```python
from build123d import *

# Parameters (mm, degrees)
SKETCH1_R           = 75
BOSS_EXTRUDE1_DEPTH = 20
BOSS_EXTRUDE2_DEPTH = 7.5
BOSS_EXTRUDE3_START = 7.5
SKETCH2_4_R         = 2.25
BOSS_EXTRUDE3_DEPTH = 20
BOSS_EXTRUDE4_START = -22.5
SKETCH2_5_R         = 2.25
BOSS_EXTRUDE4_DEPTH = 15


with BuildPart() as part:
    # Sketch1 → Boss-Extrude1 (new body)
    with BuildSketch(Plane(origin=(0, 0, 0), x_dir=(1, 0, 0), z_dir=(0, 1, 0))):
        with Locations(Location((0, 0, 0), (0, 0, 270))):
            Circle(SKETCH1_R)
    extrude(amount=BOSS_EXTRUDE1_DEPTH)

    # Sketch2 → Boss-Extrude2 (add, symmetric)
    with BuildSketch(Plane.XY):
        Polygon((75, 20), (-75, 20), (-117.25, 55), (0, 55), (75, 60), align=None)
    extrude(amount=BOSS_EXTRUDE2_DEPTH, both=True)

    # Sketch2<4> → Boss-Extrude3 (add)
    # profile 1 of 2: a face of its own
    with BuildSketch(Plane.XY.offset(BOSS_EXTRUDE3_START)):
        Polygon((-75, 20), (75, 20), (75, 60), (0, 55), (-117.25, 55), align=None)
    # profile 2 of 2: a face of its own
    with BuildSketch(Plane.XY.offset(BOSS_EXTRUDE3_START)):
        Polygon((0, 55), (75, 60), (-65, 90), (-65, 170), (-117.25, 170), (-117.25, 55), align=None)
        with Locations((-95, 80)):
            Circle(SKETCH2_4_R, mode=Mode.SUBTRACT)
        with Locations((-95, 150)):
            Circle(SKETCH2_4_R, mode=Mode.SUBTRACT)
    extrude(amount=BOSS_EXTRUDE3_DEPTH)

    # Sketch2<5> → Boss-Extrude4 (add)
    with BuildSketch(Plane.XY.offset(BOSS_EXTRUDE4_START)):
        Polygon((75, 20), (-75, 20), (-117.25, 55), (-117.25, 170), (-65, 170), (-65, 90), (75, 60), align=None)
        with Locations((-95, 150)):
            Circle(SKETCH2_5_R, mode=Mode.SUBTRACT)
        with Locations((-95, 80)):
            Circle(SKETCH2_5_R, mode=Mode.SUBTRACT)
    extrude(amount=BOSS_EXTRUDE4_DEPTH)


solid = part.part
```
Here's how the part is built. I have some questions about the finished solid (model axes, mm). A direction names the side the tool comes from. Give positions to 0.01 mm unless a question says otherwise; leave off trailing zeros. Write each loop counter-clockwise with the first axis right and the second up, starting at its lowest first coordinate (ties: lowest second). Pieces come first, ordered by that corner, then holes.
(1) Will these pins go through, and if not, where does the flat tip stop? pin 1 (1.5 mm diameter, centred on x = -63.5, y = 72, fed in from +Z); pin 2 (6 mm diameter, centred on y = 120.5, z = 15, fed in from +X); pin 3 (4 mm diameter, centred on x = -85.5, y = 135.5, fed in from -Z).
Output values:
pin 1: stops at z = 27.5
pin 2: stops at x = -65
pin 3: stops at z = -22.5
(2) Imagine slicing it at D-D, the plane x = -49. Write out the boundary of the cut face in (y, z).
Output values:
outline: (0, -56.78) - (20, -56.78) - (20, -22.5) - (86.57, -22.5) - (86.57, -7.5) - (55, -7.5) - (55, 7.5) - (86.57, 7.5) - (86.57, 27.5) - (20, 27.5) - (20, 56.78) - (0, 56.78) - close
(3) If I drill on L1, parallel to Z at x = -54.5, y = 77; L2, parallel to X at y = 150, z = -13.5; L3, parallel to Y at x = -95, z = 12, over which ranges is the centre line in solid material (lowest first)?
Output values:
L1: z = -22.5 to -7.5, 7.5 to 27.5
L2: x = -117.25 to -97.25, -92.75 to -65
L3: y = 36.57 to 77.75, 82.25 to 147.75, 152.25 to 170
(4) On a 3-axis mill with a long thin cutter (end or side, diameter ignored), from which of +Z, -Z, +X, -X, +Y, -Y can I reach the whole of each face in a straight line? I mean faces 1 (the face through (73, 20, 20)), 2 (the face through (-65, 131, -15)), 3 (the face through (1, 20, 46)), 4 (the face through (-45.636, 9.86, -59.517)), 5 (the face through (-41, 79, -22.5)). Say none if no direction works.
Output values:
face 1: +Z, +X, -Y
face 2: +Z, -Z, +X, +Y
face 3: +Z, +X, -X, +Y
face 4: -Y
face 5: -Z, +X, -X, +Y
(5) Imagine slicing it at C-C, the plane y = 41. Write out the boundary of the cut face in (x, z).
Output values:
outline: (-100.35, -22.5) - (75, -22.5) - (75, 27.5) - (-100.35, 27.5) - close
(6) Imagine slicing it at B-B, the plane z = 23. Write out the boundary of the cut face in (x, y), and give its area (3 significant figures).
Output values:
outline: (-117.25, 55) - (-75, 20) - (-71.39, 20) - (-71.39, 0) - (71.39, 0) - (71.39, 20) - (75, 20) - (75, 60) - (-65, 90) - (-65, 170) - (-117.25, 170) - close; hole circle Ø4.5 at (-95, 80); hole circle Ø4.5 at (-95, 150)
area: 17,600 mm2
(7) Thinking about a two-plate mould opening in Y: for faces 6 (the face through (-92.92, 149.14, 17.36)), 7 (the face through (-71, 104, -7.5)), 8 (the face through (-92.92, 79.14, 17.36)), 9 (the face through (5.98, 74.79, 17.36)), which applies, pulls with the +Y half, pulls with the -Y half, needs draft (parallel to the pull), parting line crosses it, or undercut?
Output values:
face 6: undercut
face 7: needs draft
face 8: undercut
face 9: pulls with the +Y half
(8) Imagine slicing it at A-A, the plane y = 133.5. Write out the boundary of the cut face in (x, z).
Output values:
outline: (-117.25, -22.5) - (-65, -22.5) - (-65, -7.5) - (-117.25, -7.5) - close; (-117.25, 7.5) - (-65, 7.5) - (-65, 27.5) - (-117.25, 27.5) - close
